Build history of the part. All positions in model axes, mm. A direction names the side the tool comes from. Round coordinates to 2 decimals unless told otherwise and drop trailing zeros. Order: outer loops, then holes, each group sorted by start corner. A loop starts at its lowest first (then second) coordinate and runs counter-clockwise, first axis right, second up. Notation, with made-up numbers: (-39.75, 86) -> (13.25, 86) arc R16 cw to (13.25, 95) -> close; hole circle Ø7 at (-9.5, 49.5). An arc over 180 degrees is marked (long way). Write item = value, one per line.
from build123d import *

# Parameters (mm, degrees)
F1_DEPTH = 95
F2_R     = 1.5
F3_DEPTH = 5


with BuildPart() as f1:
    # F0 (on Top) → F1 (new body)
    with BuildSketch(Plane.XY):
        Polygon((36.5, 0), (0, 0), (-36.5, 0), (-36.5, -18), (-34.5, -18), (-34.5, -5), (-24.5, -5), (-24.5, -18), (-22.5, -18), (-22.5, -5), (-12.5, -5), (-12.5, -18), (-10.5, -18), (-10.5, -5), (0, -5), (10.5, -5), (10.5, -18), (12.5, -18), (12.5, -5), (22.5, -5), (22.5, -18), (24.5, -18), (24.5, -5), (34.5, -5), (34.5, -18), (36.5, -18), align=None)
    extrude(amount=F1_DEPTH)

    # F2 (on face) → F3 (cut, through all)
    with BuildSketch(Plane.XZ.offset(5)):
        with Locations((0, 85)):
            Circle(F2_R)
        with Locations((0, 47.5)):
            Circle(F2_R)
        with Locations((0, 10)):
            Circle(F2_R)
    extrude(amount=-F3_DEPTH, mode=Mode.SUBTRACT)


solid = f1.part
Q1. Cut at B-B, the plane y = -6.5. List the corners of the cut face in (x, z).
Check values:
outline = (-36.5, 0) -> (-34.5, 0) -> (-34.5, 95) -> (-36.5, 95) -> close; (-24.5, 0) -> (-22.5, 0) -> (-22.5, 95) -> (-24.5, 95) -> close; (-12.5, 0) -> (-10.5, 0) -> (-10.5, 95) -> (-12.5, 95) -> close; (10.5, 0) -> (12.5, 0) -> (12.5, 95) -> (10.5, 95) -> close; (22.5, 0) -> (24.5, 0) -> (24.5, 95) -> (22.5, 95) -> close; (34.5, 0) -> (36.5, 0) -> (36.5, 95) -> (34.5, 95) -> close
Q2. Cut at A-A, the plane x = 0. List the corners of the cut face in (y, z).
Check values:
outline = (-5, 0) -> (0, 0) -> (0, 8.5) -> (-5, 8.5) -> close; (-5, 11.5) -> (0, 11.5) -> (0, 46) -> (-5, 46) -> close; (-5, 49) -> (0, 49) -> (0, 83.5) -> (-5, 83.5) -> close; (-5, 86.5) -> (0, 86.5) -> (0, 95) -> (-5, 95) -> close
Q3. Which spindle directions (+Z, -Z, +X, -X, +Y, -Y) get a long thin tool onto all of the face, cutting with end or side? Do faces 1 (the face through (12.5, -12, 47)), 2 (the face through (0, -3, 46)). Say none if no direction does.
Check values:
face_1 = +Z, -Z, -Y
face_2 = +Y, -Y
Q4. Mould opens along X. For faces 3 (the face through (10.5, -11, 47)), 4 (the face through (-24, -18, 47)) say: released by +X, released by -X, zero draft, split by the parting line, or undercut.
Check values:
face_3 = undercut
face_4 = zero draft
Q5. Cut at C-C, the plane z = 47.5. List the corners of the cut face in (x, y).
Check values:
outline = (-36.5, -18) -> (-34.5, -18) -> (-34.5, -5) -> (-24.5, -5) -> (-24.5, -18) -> (-22.5, -18) -> (-22.5, -5) -> (-12.5, -5) -> (-12.5, -18) -> (-10.5, -18) -> (-10.5, -5) -> (-1.5, -5) -> (-1.5, 0) -> (-36.5, 0) -> close; (1.5, -5) -> (10.5, -5) -> (10.5, -18) -> (12.5, -18) -> (12.5, -5) -> (22.5, -5) -> (22.5, -18) -> (24.5, -18) -> (24.5, -5) -> (34.5, -5) -> (34.5, -18) -> (36.5, -18) -> (36.5, 0) -> (1.5, 0) -> close
Q6. Cut at D-D, the plane z = 80. List the corners of the cut face in (x, y).
Check values:
outline = (-36.5, -18) -> (-34.5, -18) -> (-34.5, -5) -> (-24.5, -5) -> (-24.5, -18) -> (-22.5, -18) -> (-22.5, -5) -> (-12.5, -5) -> (-12.5, -18) -> (-10.5, -18) -> (-10.5, -5) -> (10.5, -5) -> (10.5, -18) -> (12.5, -18) -> (12.5, -5) -> (22.5, -5) -> (22.5, -18) -> (24.5, -18) -> (24.5, -5) -> (34.5, -5) -> (34.5, -18) -> (36.5, -18) -> (36.5, 0) -> (-36.5, 0) -> close
Q7. Flat gauge pins, fed straight in: pin 1 (3 mm diameter, centred on x = 31.5, z = 66.5, fed in from -Y); pin 2 (2 mm diameter, centred on x = 22, y = -13.5, fed in from +Z). Where does each tip first touch, or does it go through?
Check values:
pin_1 = -5
pin_2 = 95
Q8. Probe probe 1 along X at (y, z) = (-7.5, 23.5); probe 2 along Z at (x, y) = (0, -1.25); probe 3 along X at (y, z) = (-2.75, 85). List the from-to ranges inside material, lowest first.
Check values:
probe_1 = -36.5 to -34.5, -24.5 to -22.5, -12.5 to -10.5, 10.5 to 12.5, 22.5 to 24.5, 34.5 to 36.5
probe_2 = 0 to 8.5, 11.5 to 46, 49 to 83.5, 86.5 to 95
probe_3 = -36.5 to -1.5, 1.5 to 36.5
